Autodesk Inventor part; units mm, degrees
ref_plane "Work Plane1" through (0, 0, 27) normal (0, 0, 1) x (1, 0, 0)
ref_plane "YZ Plane" through (0, 0, 0) normal (1, 0, 0) x (0, 1, 0)
ref_plane "XZ Plane" through (0, 0, 0) normal (0, 1, 0) x (-1, 0, 0)
sketch "Sketch1" plane through (0, 0, 0) normal (0, 0, 1) x (1, 0, 0)
  arc A0 (5.6974, 0.1712) -> (4.4165, -3.6034) centre (0, 0) ccw
  line L0 (37.7409, -2.5) -> (6.7409, -2.5)
  arc A1 (3.6983, 0.1111) -> (2.8668, -2.3391) centre (0, 0) ccw
  line L1 (6.7409, -0.5) -> (37.7409, -0.5)
  line L2 (37.7409, -0.5) -> (37.7409, -2.5)
  arc A2 (6.7409, -2.5) -> (4.4165, -3.6034) centre (6.7409, -5.5) ccw
  arc A3 (6.7409, -0.5) -> (2.8668, -2.3391) centre (6.7409, -5.5) ccw
  line L3 (3.6983, 0.1111) -> (5.6974, 0.1712)
  point P0 (5.1225, -2.5)
  dimension "d0" = 11.4
  dimension "d1" = 2
  dimension "d2" = 3
  dimension "d3" = 5
  dimension "d4" = 2
  dimension "d5" = 31
  dimension "d8" = 0.5
  dimension "d9" = 0.7
extrude "Extrusion1" add sketch "Sketch1" along normal mid plane 101.6
ref_plane "Work Plane1" through (0, 0, 27) normal (0, 0, 1) x (1, 0, 0)
sketch "Sketch2" plane through (0, 0, 27) normal (0, 0, 1) x (1, 0, 0)
  arc A0 (6.7409, -2.5) -> (4.4165, -3.6034) centre (6.7409, -5.5) ccw
  arc A1 (5.6974, 0.1712) -> (4.4165, -3.6034) centre (0, 0) ccw
  line L0 (5.6974, 0.1712) -> (3.6983, 0.1111)
  arc A2 (3.6983, 0.1111) -> (2.8668, -2.3391) centre (0, 0) ccw
  arc A3 (6.7409, -0.5) -> (2.8668, -2.3391) centre (6.7409, -5.5) ccw
  line L1 (6.7409, -0.5) -> (37.7409, -0.5) construction
  line L2 (37.7409, -0.5) -> (37.7409, -2.5) construction
  line L3 (37.7409, -2.5) -> (6.7409, -2.5) construction
  line L4 (6.7409, -0.5) -> (6.7409, -2.5)
extrude "Extrusion2" cut sketch "Sketch2" along normal through all
mirror "Mirror1" about plane through (0, 0, 0) normal (0, 0, 1) of "Extrusion2"
sketch "Sketch3" plane through (0, 0, 0) normal (0, 0, 1) x (1, 0, 0)
  arc A0 (6.7409, -0.5) -> (2.8668, -2.3391) centre (6.7409, -5.5) ccw
  line L0 (6.7409, -0.5) -> (37.7409, -0.5) construction
  line L1 (37.7409, -0.5) -> (37.7409, -2.5)
  line L2 (37.7409, -2.5) -> (6.7409, -2.5) construction
  arc A1 (6.7409, -2.5) -> (4.4165, -3.6034) centre (6.7409, -5.5) ccw
  arc A2 (5.6974, 0.1712) -> (4.4165, -3.6034) centre (0, 0) ccw
  line L3 (5.6974, 0.1712) -> (3.6983, 0.1111)
  arc A3 (3.6983, 0.1111) -> (2.8668, -2.3391) centre (0, 0) ccw
  line L4 (6.7409, -2.5) -> (6.7409, -0.5)
  line L5 (6.7409, -2.5) -> (6.7409, -0.5)
extrude "Extrusion3" cut sketch "Sketch3" along normal mid plane 18.1
equation "\"d1\" = d4"
equation "\"d3\" = d2 + d4"
properties part number "HINGE PLATE 2" material "Stainless Steel"
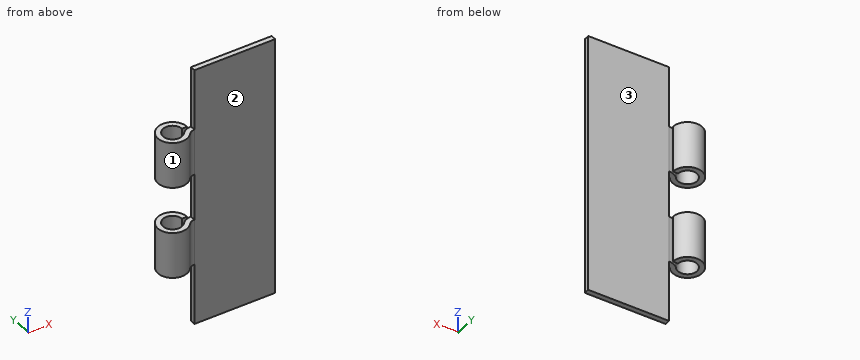
Geometry check sheet. Reference: the model listing, model coordinates, mm. Face numbers are marked on the shaded views. A direction names the side the tool comes from. Round coordinates to 2 decimals unless told otherwise and drop trailing zeros. Loops run counter-clockwise (first coordinate to the right, second up) from the corner with the lowest first, then second, coordinate; pieces in that order, holes last. Notation, with made-up numbers: (18.25, 46) - (40.25, 46) arc R27 ccw to (40.25, 66) - close; hole circle Ø5 at (70.25, 44.5). An arc over 180 degrees is marked (long way). Use a Markdown table: item, result.
Q1. Material ranges on line 1 (Y direction, x = 9.5, z = 13); line 2 (Z direction, x = 3, y = -2.25); line 3 (X direction, y = -1.5, z = 17), recorded low to high.
Solutions:
| item | result |
|---|---|
| line 1 | y = -2.5 to -0.5 |
| line 2 | z = -27 to -9.05, 9.05 to 27 |
| line 3 | x = -5.5 to -3.38, 3.74 to 37.74 |
Q2. Cross-section at A-A on y = 1.5. Record the cut outline in (x, z).
Solutions:
| item | result |
|---|---|
| outline | (-5.5, -27) - (-3.38, -27) - (-3.38, -9.05) - (-5.5, -9.05) - close; (-5.5, 9.05) - (-3.38, 9.05) - (-3.38, 27) - (-5.5, 27) - close; (3.38, -27) - (5.5, -27) - (5.5, -9.05) - (3.38, -9.05) - close; (3.38, 9.05) - (5.5, 9.05) - (5.5, 27) - (3.38, 27) - close |
Q3. Cross-section at C-C on x = 32. Record the cut outline in (y, z).
Solutions:
| item | result |
|---|---|
| outline | (-2.5, -50.8) - (-0.5, -50.8) - (-0.5, 50.8) - (-2.5, 50.8) - close |
Q4. Cross-section at B-B on z = 13. Record the cut outline in (x, y), plus the area to 3 significant figures.
Solutions:
| item | result |
|---|---|
| outline | (2.87, -2.34) arc R3.7 cw (long way) to (3.7, 0.11) - (5.7, 0.17) arc R5.7 ccw (long way) to (4.42, -3.6) arc R3 cw to (6.74, -2.5) - (37.74, -2.5) - (37.74, -0.5) - (6.74, -0.5) arc R5 ccw to start |
| area | 121 mm2 |
Q5. Go/stop test with flat-tipped pins: P1, Ø0.6, axis at y = -2, z = 38.5, coming from the -X side; P2, Ø3.5, axis at x = 1.5, y = -1, coming from the -Z side; P3, Ø4, axis at x = 33, z = 10, coming from the +Y side; P4, Ø9.5, axis at x = 18.5, z = -2.5, coming from the -Y side. Record where each tip stops, or that it passes through.
Solutions:
| item | result |
|---|---|
| P1 | stops at x = 6.74 |
| P2 | passes through |
| P3 | stops at y = -0.5 |
| P4 | stops at y = -2.5 |
Q6. Access from +Z, -Z, +X, -X, +Y, -Y to the whole of each face (thin tool, end or side, straight path). Record for the marked faces 1, 2 and 3.
Solutions:
| item | result |
|---|---|
| face 1 | +Z, -Z |
| face 2 | +Z, -Z, +X, -Y |
| face 3 | +Z, -Z, +X, +Y |
